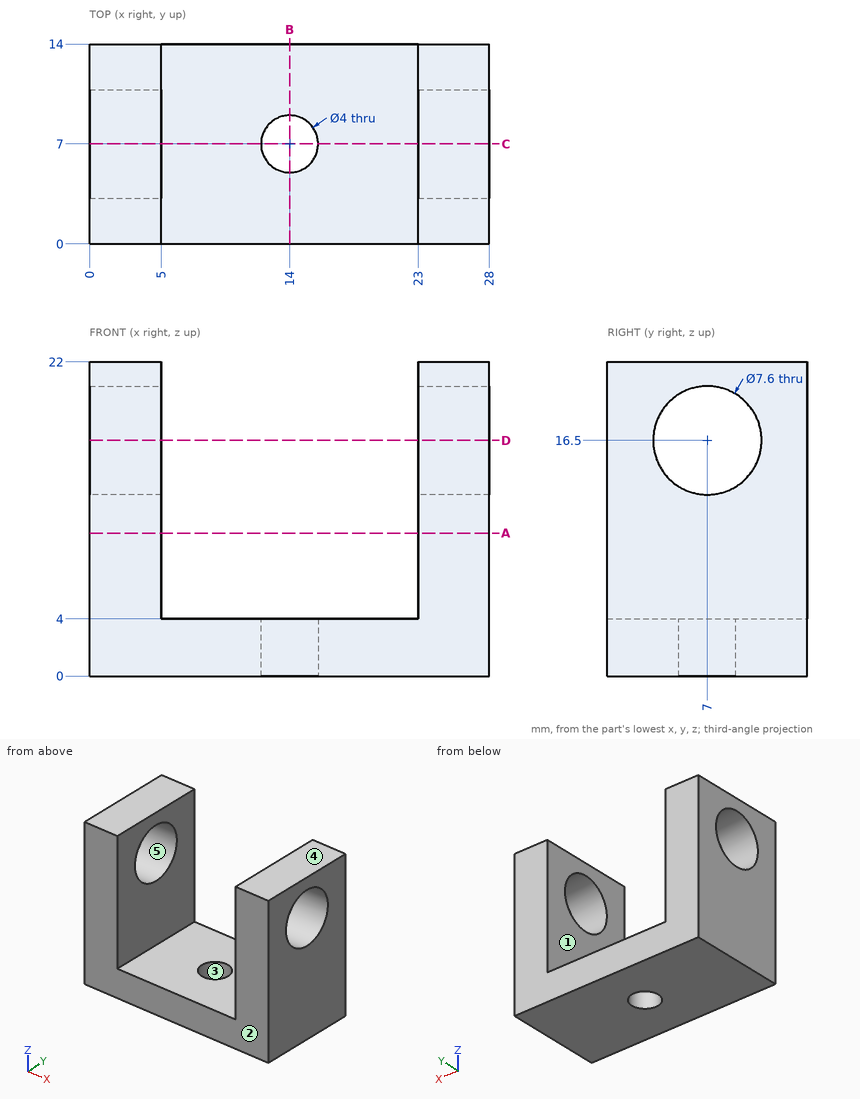
Could you check a few things on this drawing? It's one solid part, dimensions in mm from its lowest x, y, z. A direction names the side the tool comes from. Coordinates: 2 decimals unless noted, no trailing zeros. Order: outer loops, then holes, each group sorted by start corner. A loop starts at its lowest first (then second) coordinate and runs counter-clockwise, first axis right, second up. Notation, with made-up numbers: M -8,78.5 L 41,78.5 A28 ccw 41,108.5 Z; hole C 50,3.25 d3. An arc over 180 degrees is marked long. Use a Markdown table: item, result. Add a question column.
Q1. I want a section at B-B on x = 14. List the corners of the cut face in (y, z) for me, then the cut area to 3 significant figures.
Q2. I want a section at A-A on z = 10. List the corners of the cut face in (x, y) for me, then the cut area to 3 significant figures.
Q3. If I drill on L1, parallel to X at y = 6, z = 21; L2, parallel to Y at x = 3.25, z = 16.25; L3, parallel to Y at x = 14, z = 2.4, over which ranges is the centre line in solid material (lowest first)?
Q4. I want a section at C-C on y = 7. List the corners of the cut face in (x, z) for me, then the cut area to 3 significant figures.
Q5. I want a section at D-D on z = 16.5. List the corners of the cut face in (x, y) for me.
Q6. Which directions (+Z, -Z, +X, -X, +Y, -Y) give clear straight access to the entire face, cutting with the end or side of a thin tool? Please do the marked faces 1 and 2.
Q7. We'd pull the mould along Z, two halves only. Please class the marked faces 3, 4 and 5: pulls with the +Z half, pulls with the -Z half, needs draft (parallel to the pull), parting line crosses it, or undercut.
Q8. I'm going to push flat-ended pins straight in: pin 1 (2.5 mm diameter, centred on x = 14, y = 7, fed in from -Z); pin 2 (1 mm diameter, centred on x = 16, y = 10, fed in from -Z); pin 3 (4 mm diameter, centred on x = 11.5, y = 5, fed in from +Z). Where does each tip first touch, or does it pass through?
Checked values:
| question | item | result |
|---|---|---|
| 1 | outline | M 0,0 L 5,0 L 5,4 L 0,4 Z; M 9,0 L 14,0 L 14,4 L 9,4 Z |
| 1 | area | 40.0 mm² |
| 2 | outline | M 0,0 L 5,0 L 5,14 L 0,14 Z; M 23,0 L 28,0 L 28,14 L 23,14 Z |
| 2 | area | 140 mm² |
| 3 | L1 | 0 to 5, 23 to 28 |
| 3 | L2 | 0 to 3.21, 10.79 to 14 |
| 3 | L3 | 0 to 5, 9 to 14 |
| 4 | outline | M 0,0 L 12,0 L 12,4 L 5,4 L 5,12.7 L 0,12.7 Z; M 0,20.3 L 5,20.3 L 5,22 L 0,22 Z; M 16,0 L 28,0 L 28,12.7 L 23,12.7 L 23,4 L 16,4 Z; M 23,20.3 L 28,20.3 L 28,22 L 23,22 Z |
| 4 | area | 200 mm² |
| 5 | outline | M 0,0 L 5,0 L 5,3.2 L 0,3.2 Z; M 0,10.8 L 5,10.8 L 5,14 L 0,14 Z; M 23,0 L 28,0 L 28,3.2 L 23,3.2 Z; M 23,10.8 L 28,10.8 L 28,14 L 23,14 Z |
| 6 | face 1 | +Z, +Y, -Y |
| 6 | face 2 | +Z, -Z, +X, -X, -Y |
| 7 | face 3 | needs draft |
| 7 | face 4 | pulls with the +Z half |
| 7 | face 5 | undercut |
| 8 | pin 1 | through |
| 8 | pin 2 | z = 0 |
| 8 | pin 3 | z = 4 |
